Read the model definition and answer for the solid it produces. Units are mm, in the model's axes. A direction names the side the tool comes from. Coordinates: 2 decimals unless noted, no trailing zeros. Order: outer loops, then holes, each group sorted by start corner. A loop starts at its lowest first (then second) coordinate and runs counter-clockwise, first axis right, second up. Notation, with made-up numbers: (-19, 60) - (0, 60) arc R21 ccw to (0, 84) - close; hole circle Ø8 at (76, 65). An arc over 180 degrees is marked (long way). Use one line per item in the form item = value.
```python
from build123d import *

# Parameters (mm, degrees)
SKETCH_1_W          = 20
SKETCH_1_H          = 20
EXTRUDE_1_DEPTH     = 130
SKETCH_2_W          = 5.996199515
SKETCH_2_H          = 130
CUT_EXTRUDE_1_DEPTH = 4.5
HOLE_WIZARD_M5_1_D  = 4.2
SKETCH_5_R          = 2.5
CUT_EXTRUDE_2_DEPTH = 21


with BuildPart() as part:
    # 草图1 → 凸台-拉伸1 (new body)
    with BuildSketch(Plane.XY):
        with Locations((10, 10)):
            Rectangle(SKETCH_1_W, SKETCH_1_H)
    extrude(amount=EXTRUDE_1_DEPTH)

    # 草图2 → 切除-拉伸1 (cut)
    with BuildSketch(Plane(origin=(0, 20, 0), x_dir=(1, 0, 0), z_dir=(0, 1, 0))):
        with Locations((13.673460813, -65)):
            Rectangle(SKETCH_2_W, SKETCH_2_H)
    extrude(amount=-CUT_EXTRUDE_1_DEPTH, mode=Mode.SUBTRACT)

    # M5 螺纹孔1 (through all)
    with Locations(Plane.ZY):
        with Locations((20, 8), (50, 8)):
            Hole(HOLE_WIZARD_M5_1_D / 2)

    # 草图5 → 切除-拉伸2 (cut, through all)
    with BuildSketch(Plane(origin=(20, 0, 0), x_dir=(0, 0, -1), z_dir=(1, 0, 0))):
        with Locations((-35, 8)):
            Circle(SKETCH_5_R)
    extrude(amount=-CUT_EXTRUDE_2_DEPTH, mode=Mode.SUBTRACT)


solid = part.part
```
(1) Which of the six approach directions +Z, -Z, +X, -X, +Y, -Y give full straight-line access (tool end or side, diameter ignored) to faces 1 (the flat face through (10, 10, 130)), 2 (the flat face through (16.672, 18, 66))?
Answer list:
face_1 = +Z, +X, -X, +Y, -Y
face_2 = +Z, -Z, +Y
(2) Section A-A, the plane x = 1.5 is taken. Write down the section's boundary in (y, z).
Answer list:
outline = (0, 0) - (20, 0) - (20, 130) - (0, 130) - close; hole circle Ø5 at (8, 35); hole circle Ø4.2 at (8, 20); hole circle Ø4.2 at (8, 50)
(3) Straight lines are drawn through the part: L1, parallel to X at y = 17, z = 54; L2, parallel to Y at x = 9.25, z = 35; L3, parallel to Y at x = 6.25, z = 50. For each, find the intervals that lie inside material, in ascending order.
Answer list:
L1 = 0 to 10.68, 16.67 to 20
L2 = 0 to 5.5, 10.5 to 20
L3 = 0 to 5.9, 10.1 to 20
(4) Given pin 1 Ø1.5 at (x, z) = (15, 26) entering from +Y; pin 2 Ø4 at (y, z) = (8, 20) entering from +X, each flat-ended and moving along its own axis, determine where each tip first touches the part or whether it passes through.
Answer list:
pin_1 = 15.5
pin_2 = through
(5) Section C-C, the plane y = 17.5 is taken. Write down the section's boundary in (x, z).
Answer list:
outline = (0, 0) - (10.68, 0) - (10.68, 130) - (0, 130) - close; (16.67, 0) - (20, 0) - (20, 130) - (16.67, 130) - close
(6) Section B-B, the plane z = 20 is taken. Write down the section's boundary in (x, y).
Answer list:
outline = (0, 0) - (20, 0) - (20, 5.9) - (0, 5.9) - close; (0, 10.1) - (20, 10.1) - (20, 20) - (16.67, 20) - (16.67, 15.5) - (10.68, 15.5) - (10.68, 20) - (0, 20) - close
(7) The mould has two halves that part along Y. Classify faces 3 (the flat face through (10.675, 18, 66)), 4 (the flat face through (14, 15.5, 64)), 5 (the cylindrical face through (10.14, 9.77, 48.87)), 6 (the cylindrical face through (10.14, 7.04, 32.69)): +Y half, -Y half, draft (parallel to the pull), parting line (faces both ways), or undercut.
Answer list:
face_3 = draft
face_4 = +Y half
face_5 = undercut
face_6 = undercut
(8) Section D-D, the plane z = 35 is taken. Write down the section's boundary in (x, y), then the cut area to 3 significant figures.
Answer list:
outline = (0, 0) - (20, 0) - (20, 5.5) - (0, 5.5) - close; (0, 10.5) - (20, 10.5) - (20, 20) - (16.67, 20) - (16.67, 15.5) - (10.68, 15.5) - (10.68, 20) - (0, 20) - close
area = 273 mm2
